Geometry check sheet. Reference: the model listing, model coordinates, mm. A direction names the side the tool comes from. Give positions to 0.01 mm unless a question says otherwise; leave off trailing zeros. Loops run counter-clockwise (first coordinate to the right, second up) from the corner with the lowest first, then second, coordinate; pieces in that order, holes last. Notation, with made-up numbers: (62.25, 44.25) -> (92.25, 44.25) arc R34 ccw to (92.25, 76.25) -> close; hole circle Ø1 at (85, 26.25). An arc over 180 degrees is marked (long way). Write item = value, one per line.
```python
from build123d import *

# Parameters (mm, degrees)
F1_DEPTH = 25.4


with BuildPart() as f1:
    # F0 (on Front) → F1 (new body)
    with BuildSketch(Plane.XZ):
        Polygon((-1.905, 0), (0, 0), (50.8, 0), (50.8, 3.175), (50.165, 2.54), (49.53, 3.175), (48.895, 2.54), (48.26, 3.175), (47.625, 2.54), (46.99, 3.175), (46.355, 2.54), (45.72, 3.175), (45.085, 2.54), (44.45, 3.175), (43.815, 2.54), (43.18, 3.175), (42.545, 2.54), (41.91, 3.175), (41.275, 2.54), (40.64, 3.175), (40.005, 2.54), (39.37, 3.175), (38.735, 2.54), (38.1, 3.175), (37.465, 2.54), (36.83, 3.175), (36.195, 2.54), (35.56, 3.175), (34.925, 2.54), (34.29, 3.175), (33.655, 2.54), (33.02, 3.175), (32.385, 2.54), (31.75, 3.175), (31.115, 2.54), (30.48, 3.175), (29.845, 2.54), (29.21, 3.175), (28.575, 2.54), (27.94, 3.175), (27.305, 2.54), (26.67, 3.175), (26.035, 2.54), (25.4, 3.175), (24.765, 2.54), (24.13, 3.175), (23.495, 2.54), (22.86, 3.175), (22.225, 2.54), (21.59, 3.175), (20.955, 2.54), (20.32, 3.175), (19.685, 2.54), (19.05, 3.175), (18.415, 2.54), (17.78, 3.175), (17.145, 2.54), (16.51, 3.175), (15.875, 2.54), (15.24, 3.175), (14.605, 2.54), (13.97, 3.175), (13.335, 2.54), (12.7, 3.175), (12.065, 2.54), (11.43, 3.175), (10.795, 2.54), (10.16, 3.175), (9.525, 2.54), (8.89, 3.175), (8.255, 2.54), (7.62, 3.175), (6.985, 2.54), (6.35, 3.175), (5.715, 2.54), (5.08, 3.175), (4.445, 2.54), (3.81, 3.175), (3.175, 2.54), (2.54, 3.175), (0, 3.175), (0, 6.35), (-1.905, 6.35), align=None)
    extrude(amount=F1_DEPTH)


solid = f1.part
```
Item 1: Thickness scan on L1, parallel to X at y = -20.25, z = 3.5 (3 decimals); L2, parallel to Z at x = 2, y = -22.25 (3 decimals); L3, parallel to Z at x = 29, y = -14.5 (3 decimals). Record the ranges inside material, lowest first. Write a range as [from, to].
Answer:
L1 = [-1.905, 0]
L2 = [0, 3.175]
L3 = [0, 2.965]
Item 2: Tool access check on faces 1 (the flat face through (0, -13, 5)), 2 (the flat face through (-1.905, -13, 3)). Record the directions out of +Z, -Z, +X, -X, +Y, -Y that give a thin tool (end or side, any length) a straight path to the whole face; none if there is none.
Answer:
face_1 = +Z, +X, +Y, -Y
face_2 = +Z, -Z, -X, +Y, -Y
Item 3: Section check A-A, the plane z = 3.75. Record the cut outline in (x, y) (3 decimals), plus the area to 3 significant figures.
Answer:
outline = (-1.905, -25.4) -> (0, -25.4) -> (0, 0) -> (-1.905, 0) -> close
area = 48.4 mm^2
Item 4: Gauge pin test, flat ends, axial feed: pin 1 (1.5 mm diameter, centred on x = 7, y = -19.5, fed in from -Z); pin 2 (0.8 mm diameter, centred on x = 0.5, y = -14.5, fed in from +Z) (3 decimals). Record the tip position at first contact, or that the pin passes through.
Answer:
pin_1 = 0
pin_2 = 3.175
